from build123d import *

# Parameters (mm, degrees)
SKETCH1_W           = 8
SKETCH1_H           = 180
BOSS_EXTRUDE1_DEPTH = 8
SKETCH3_R           = 3
BOSS_EXTRUDE4_DEPTH = 10
SKETCH3_4_R         = 3
SKETCH3_4_W         = 8
SKETCH3_4_H         = 7
BOSS_EXTRUDE5_DEPTH = 1


with BuildPart() as part:
    # Sketch1 → Boss-Extrude1 (new body)
    with BuildSketch(Plane(origin=(0, 0, 0), x_dir=(0, 0, -1), z_dir=(1, 0, 0))):
        Rectangle(SKETCH1_W, SKETCH1_H)
    extrude(amount=BOSS_EXTRUDE1_DEPTH)

    # Sketch3 → Boss-Extrude4 (add)
    with BuildSketch(Plane(origin=(8, 0, 0), x_dir=(0, 0, -1), z_dir=(1, 0, 0))):
        with Locations(Location((-1, -75, 0), (0, 0, 180))):
            Circle(SKETCH3_R)
        with Locations((1, -50)):
            Circle(SKETCH3_R)
        with Locations(Location((-1, 50, 0), (0, 0, 180))):
            Circle(SKETCH3_R)
        with Locations((1, 75)):
            Circle(SKETCH3_R)
    extrude(amount=BOSS_EXTRUDE4_DEPTH)

    # Sketch3_4 → Boss-Extrude5 (add)
    # profile 1 of 8: a face of its own
    with BuildSketch(Plane(origin=(8, 0, 0), x_dir=(0, 0, -1), z_dir=(1, 0, 0))):
        Polygon((4, 78.5), (-4, 78.5), (-4, 71.5), (4, 71.5), (4, 75), align=None)
        with Locations((1, 75)):
            Circle(SKETCH3_4_R, mode=Mode.SUBTRACT)
    # profile 2 of 8: a face of its own
    with BuildSketch(Plane(origin=(8, 0, 0), x_dir=(0, 0, -1), z_dir=(1, 0, 0))):
        with Locations((1, 75)):
            Circle(SKETCH3_4_R)
    # profile 3 of 8: a face of its own
    with BuildSketch(Plane(origin=(8, 0, 0), x_dir=(0, 0, -1), z_dir=(1, 0, 0))):
        Polygon((4, 53.5), (-4, 53.5), (-4, 50), (-4, 46.5), (4, 46.5), align=None)
        with BuildLine():
            ThreePointArc((2, 50), (-1, 47), (-4, 50))
            ThreePointArc((-4, 50), (-1, 53), (2, 50))
        make_face(mode=Mode.SUBTRACT)
    # profile 4 of 8: a face of its own
    with BuildSketch(Plane(origin=(8, 0, 0), x_dir=(0, 0, -1), z_dir=(1, 0, 0))):
        with Locations(Location((-1, 50, 0), (0, 0, 180))):
            Circle(SKETCH3_4_R)
    # profile 5 of 8: a face of its own
    with BuildSketch(Plane(origin=(8, 0, 0), x_dir=(0, 0, -1), z_dir=(1, 0, 0))):
        Polygon((4, -50), (4, -46.5), (-4, -46.5), (-4, -53.5), (4, -53.5), align=None)
        with Locations((1, -50)):
            Circle(SKETCH3_4_R, mode=Mode.SUBTRACT)
    # profile 6 of 8: a face of its own
    with BuildSketch(Plane(origin=(8, 0, 0), x_dir=(0, 0, -1), z_dir=(1, 0, 0))):
        with Locations((1, -50)):
            Circle(SKETCH3_4_R)
    # profile 7 of 8: a face of its own
    with BuildSketch(Plane(origin=(8, 0, 0), x_dir=(0, 0, -1), z_dir=(1, 0, 0))):
        with Locations(Location((-1, -75, 0), (0, 0, 180))):
            Circle(SKETCH3_4_R)
    # profile 8 of 8: a face of its own
    with BuildSketch(Plane(origin=(8, 0, 0), x_dir=(0, 0, -1), z_dir=(1, 0, 0))):
        with Locations((0, -75)):
            Rectangle(SKETCH3_4_W, SKETCH3_4_H)
    extrude(amount=BOSS_EXTRUDE5_DEPTH)


solid = part.part
Can you work these out from the model? Positions are in its coordinate system, mm. A direction names the side the tool comes from. Coordinates: 2 decimals unless noted, no trailing zeros. Order: outer loops, then holes, each group sorted by start corner. A loop starts at its lowest first (then second) coordinate and runs counter-clockwise, first axis right, second up. Notation, with made-up numbers: (-29, -14) -> (-16, -14) arc R17 cw to (-16, 0) -> close; hole circle Ø4 at (69, 89). An arc over 180 degrees is marked (long way). Use one line per item in the form item = value.
Q1. Which directions (+Z, -Z, +X, -X, +Y, -Y) give clear straight access to the entire face, cutting with the end or side of a thin tool? Please do faces 1 (the face through (8, 63, 0)), 2 (the face through (8, 84, 0)), 3 (the face through (13, 47, 1)).
From the geometry:
face_1 = +Z, -Z, +X
face_2 = +Z, -Z, +X, +Y
face_3 = +X
Q2. I need wall thicknesses on L1, parallel to Y at x = 8.75, z = 1; L2, parallel to Y at x = 13.5, z = -0.75; L3, parallel to X at y = -30.5, z = 1.75. Which ranges of each line are inside material? Lowest first, please.
From the geometry:
L1 = -78.5 to -71.5, -53.5 to -46.5, 46.5 to 53.5, 71.5 to 78.5
L2 = -77.44 to -72.56, -52.99 to -47.01, 47.56 to 52.44, 72.01 to 77.99
L3 = 0 to 8
Q3. Will these pins go through, and if not, where does the flat tip stop? P1, Ø0.5, axis at x = 8.5, z = 1.5, coming from the -Y side; P2, Ø4, axis at y = 84, z = -1.5, coming from the +X side; P3, Ø4, axis at y = 61.5, z = 1.5, coming from the -X side; P4, Ø1, axis at x = 13.5, z = 3, coming from the +Y side.
From the geometry:
P1 = -78.5
P2 = 8
P3 = 0
P4 = 52.6
Q4. We'd pull the mould along Y, two halves only. Please class faces 4 (the face through (4, -90, 0)), 5 (the face through (9, 52, -2)), 6 (the face through (4, -1, -4)): released by +Y, released by -Y, zero draft, split by the parting line, or undercut.
From the geometry:
face_4 = released by -Y
face_5 = undercut
face_6 = zero draft
Q5. Imagine slicing it at A-A, the plane x = 10.5. List the corners of the cut face in (y, z) for me.
From the geometry:
outline = circle Ø6 at (-75, 1); circle Ø6 at (-50, -1); circle Ø6 at (50, 1); circle Ø6 at (75, -1)
Q6. Imagine slicing it at B-B, the plane y = 25. List the corners of the cut face in (x, z) for me.
From the geometry:
outline = (0, -4) -> (8, -4) -> (8, 4) -> (0, 4) -> close
